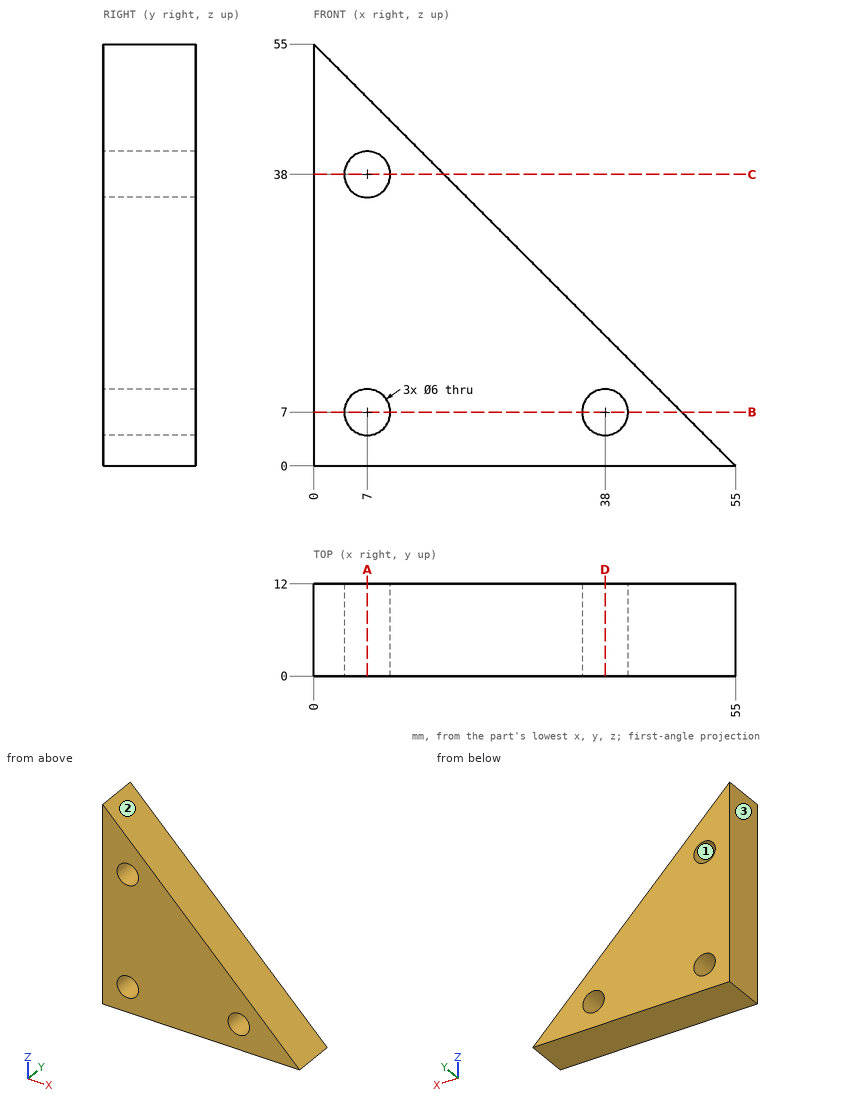
Job drawing, mm, ordinate dimensions from the low corner. One solid piece. Give positions to 0.01 mm unless a question says otherwise; leave off trailing zeros. Loops run counter-clockwise (first coordinate to the right, second up) from the corner with the lowest first, then second, coordinate; pieces in that order, holes last. Notation, with made-up numbers: M 28,34 L 42,34 A19 cw 42,52 Z; hole C -36.75,-9 d8. An arc over 180 degrees is marked long. Use one line per item in the form item = value.
Item 1: Slice it at A-A on x = 7. List the corners of the cut face in (y, z), and give its area (3 significant figures).
Filled in:
outline = M 0,0 L 12,0 L 12,4 L 0,4 Z; M 0,10 L 12,10 L 12,35 L 0,35 Z; M 0,41 L 12,41 L 12,48 L 0,48 Z
area = 432 mm^2
Item 2: Slice it at B-B on z = 7. List the corners of the cut face in (x, y), and give its area (3 significant figures).
Filled in:
outline = M 0,0 L 4,0 L 4,12 L 0,12 Z; M 10,0 L 35,0 L 35,12 L 10,12 Z; M 41,0 L 48,0 L 48,12 L 41,12 Z
area = 432 mm^2
Item 3: Slice it at C-C on z = 38. List the corners of the cut face in (x, y).
Filled in:
outline = M 0,0 L 4,0 L 4,12 L 0,12 Z; M 10,0 L 17,0 L 17,12 L 10,12 Z
Item 4: Slice it at D-D on x = 38. List the corners of the cut face in (y, z).
Filled in:
outline = M 0,0 L 12,0 L 12,4 L 0,4 Z; M 0,10 L 12,10 L 12,17 L 0,17 Z
Item 5: Drill centre lines: L1, parallel to Z at x = 7, y = 9.25; L2, parallel to X at y = 2.75, z = 8; L3, parallel to X at y = 5.5, z = 44. Where is each one in solid material? Low to high.
Filled in:
L1 = 0 to 4, 10 to 35, 41 to 48
L2 = 0 to 4.17, 9.83 to 35.17, 40.83 to 47
L3 = 0 to 11
Item 6: Flat gauge pins, fed straight in: pin 1 Ø5 at (x, z) = (38, 7) entering from +Y; pin 2 Ø6 at (y, z) = (5, 34.5) entering from +X; pin 3 Ø6 at (x, y) = (26.5, 8.5) entering from +Z; pin 4 Ø1 at (y, z) = (7.5, 28) entering from +X. Where does each tip first touch, or does it go through?
Filled in:
pin_1 = through
pin_2 = 23.5
pin_3 = 31.5
pin_4 = 27.5
Item 7: Two-plate mould, pull along Z, no slides. Class the marked faces 1, 2 and 3: released by +Z, released by -Z, zero draft, split by the parting line, or undercut.
Filled in:
face_1 = undercut
face_2 = released by +Z
face_3 = zero draft
